Autodesk Inventor part; units mm, degrees
ref_plane "YZ Plane" through (0, 0, 0) normal (1, 0, 0) x (0, 1, 0)
ref_plane "XZ Plane" through (0, 0, 0) normal (0, 1, 0) x (-1, 0, 0)
ref_plane "XY Plane" through (0, 0, 0) normal (0, 0, 1) x (1, 0, 0)
sketch "Sketch1" plane through (0, 0, 0) normal (0, 0, 1) x (1, 0, 0)
  line L0 (0, 0) -> (25, 0)
  line L1 (25, 0) -> (25, 40)
  line L2 (25, 40) -> (0, 40)
  line L3 (0, 40) -> (0, 0)
  dimension "d1" = 25
  dimension "d2" = 40
  dimension "d3" = 25
extrude "Extrusion1" add sketch "Sketch1" against normal blind 30
sketch "Sketch2" plane through (25, 0, 0) normal (1, 0, 0) x (0, 0, -1)
  line L0 (0, 0) -> (30, 0)
  circle A0 centre (15, 6.56) radius 2.46
extrude "Extrusion2" cut sketch "Sketch2" against normal blind 30
sketch "Sketch3" plane through (0, 0, 0) normal (-1, 0, 0) x (0, 0, 1)
  line L0 (0, 0) -> (-30, 0)
  line L1 (-25.05, 0) -> (-4.95, 0)
  line L2 (-4.95, 0) -> (-4.95, 33.12)
  line L3 (-4.95, 33.12) -> (-25.05, 33.12)
  line L4 (-25.05, 33.12) -> (-25.05, 0)
  dimension "d11" = 20.1
extrude "Extrusion3" cut sketch "Sketch3" against normal blind 20
sketch "Sketch4" plane through (0, 0, 0) normal (0, -1, 0) x (1, 0, 0)
  line L0 (20, -4.95) -> (20, -25.05)
  line L1 (20, -15) -> (25, -15)
  line L2 (25, 0) -> (25, -30)
  line L3 (20, -8.025) -> (25, -8.025)
  line L4 (25, -8.025) -> (25, -21.975)
  line L5 (25, -21.975) -> (20, -21.975)
  line L6 (20, -21.975) -> (20, -8.025)
  line L7 (20, -8.025) -> (25, -21.975) construction
  line L8 (25, -8.025) -> (20, -21.975) construction
  line L9 (25, -12.54) -> (25, -17.46)
  point P0 (0, 0)
  point P1 (22.5, -15)
  dimension "d14" = 13.95
extrude "Extrusion4" add sketch "Sketch4" along normal blind 15
sketch "Sketch5" plane through (20, 0, 0) normal (-1, 0, 0) x (0, 0, 1)
  circle A0 centre (-15, 6.56) radius 2.46
  circle A1 centre (-15, 6.56) radius 4.7025
  circle A2 centre (-15, 6.56) radius 2.46
  circle A3 centre (-15, 6.56) radius 2.46
  point P0 (0, 0)
  dimension "d17" = 9.405
extrude "Extrusion5" cut sketch "Sketch5" against normal blind 2.1
sketch "Sketch6" plane through (25, 0, 0) normal (1, 0, 0) x (0, 0, -1)
  circle A0 centre (15, 6.56) radius 4.7025
  line L0 (15, 6.56) -> (15, 23.56)
  circle A1 centre (15, 23.56) radius 2.46
  point P0 (0, 0)
  dimension "d20" = 17
  dimension "d21" = 4.92
extrude "Extrusion6" cut sketch "Sketch6" against normal blind 10 contours A1
sketch "Sketch7" plane through (20, 0, 0) normal (-1, 0, 0) x (0, 0, 1)
  circle A0 centre (-15, 23.56) radius 2.46
  circle A1 centre (-15, 23.56) radius 4.7025
  point P0 (0, 0)
  dimension "d24" = 9.405
extrude "Extrusion7" cut sketch "Sketch7" against normal blind 2.1
sketch "Sketch9" plane through (25, 0, 0) normal (1, 0, 0) x (0, 0, -1)
  circle A0 centre (15, 6.56) radius 2.46
  circle A1 centre (15, 6.56) radius 2.46
  circle A2 centre (15, 23.56) radius 2.46
  circle A3 centre (15, 23.56) radius 2.46
  line L0 (30, 40) -> (30, 0)
  line L1 (30, 0) -> (30, 40)
  line L2 (30, 40) -> (0, 40)
  line L3 (0, 40) -> (0, 0)
  line L4 (0, 0) -> (8.025, 0)
  line L5 (21.975, 0) -> (21.975, -15)
  line L6 (21.975, -15) -> (8.025, -15)
  line L7 (8.025, -15) -> (8.025, 0)
  line L8 (0, 0) -> (8.025, 0)
  line L9 (21.975, 0) -> (30, 0)
extrude "Extrusion8" add sketch "Sketch9" along normal blind 5
sketch "Sketch10" plane through (0, 40, 0) normal (0, 1, 0) x (1, 0, 0)
  line L0 (0, 30) -> (30, 30)
  line L1 (30, 0) -> (0, 0)
  line L2 (0, 30) -> (30, 30)
  line L3 (30, 30) -> (30, 0)
  line L4 (30, 0) -> (0, 0)
  line L5 (0, 0) -> (0, 30)
extrude "Extrusion9" add sketch "Sketch10" along normal blind 30
sketch "Sketch12" plane through (30, 0, 0) normal (1, 0, 0) x (0, 0, -1)
  circle A0 centre (15, 6.56) radius 2.46
  line L0 (15, 6.56) -> (15, 15.06)
  circle A1 centre (15, 15.06) radius 2.525
  point P0 (0, 0)
  dimension "d31" = 8.5
  dimension "d33" = 5.05
extrude "Extrusion10" cut sketch "Sketch12" against normal blind 30 contours A1
sketch "Sketch14" plane through (0, 0, 0) normal (0, 0, 1) x (1, 0, 0)
  line L0 (30, 70) -> (0, 70)
  line L1 (0, 70) -> (0, 85)
  line L2 (-15, 100) -> (-23, 100)
  line L3 (30, 0) -> (30, 70)
  line L4 (30, 113) -> (30, 70)
  arc A0 (0, 85) -> (-15, 100) centre (-15, 85) ccw
  line L5 (30, 105) -> (30, 100)
  line L6 (-23, 128) -> (15, 128)
  line L7 (30, 113) -> (15, 128)
  line L8 (-23, 128) -> (-23, 100)
  point P0 (0, 0)
  point P1 (0, 100)
  dimension "d47" = 30
  dimension "d54" = 15
  dimension "d69" = 28
extrude "Extrusion12" add sketch "Sketch14" against normal blind 30
sketch "Sketch15" plane through (0, 0, -25.05) normal (-1, 0, 0) x (0, 0, 1)
  line L0 (0, 33.12) -> (20.1, 33.12)
  line L1 (20.1, 33.12) -> (20.1, 0)
  line L2 (0, 33.12) -> (20.1, 33.12)
  line L3 (20.1, 33.12) -> (20.1, 31.1)
  line L4 (20.1, 31.1) -> (0, 31.1)
  line L5 (0, 31.1) -> (0, 33.12)
  point P0 (25.05, 0)
  dimension "d57" = 2.02
extrude "Extrusion13" add sketch "Sketch15" against normal blind 20
sketch "Sketch23" plane through (-23, 128, 0) normal (0, 1, 0) x (1, 0, 0)
  line L0 (0, 0) -> (0, 30)
  line L1 (0, 15) -> (0, 2.5)
  line L2 (0, 27.5) -> (0, 15)
  line L3 (0, 27.5) -> (5, 15)
  line L4 (5, 15) -> (0, 2.5)
  point P0 (23, 0)
  dimension "d87" = 12.5
extrude "Extrusion16" cut sketch "Sketch23" against normal through all
properties part number "orien_b_20mm"
Model file for the job. Use its own axes, mm. A direction names the side the tool comes from. Give positions to 0.01 mm unless a question says otherwise; leave off trailing zeros. Loops run counter-clockwise (first coordinate to the right, second up) from the corner with the lowest first, then second, coordinate; pieces in that order, holes last. Notation, with made-up numbers: (33, 31) -> (40, 31) arc R20 ccw to (40, 59) -> close; hole circle Ø8 at (36.5, 11). An arc over 180 degrees is marked (long way). Use a Markdown table: item, result. Add a question column.
(1) Slice it at A-A on y = 15.06. List the corners of the cut face in (x, z) (3 decimals), and give its area (4 significant figures).
(2) Drop flat-ended pins along their axis: pin 1 Ø15 at (y, z) = (35.5, -14.5) entering from -X; pin 2 Ø11 at (x, y) = (24.5, -7.5) entering from -Z (3 decimals); pin 3 Ø2.5 at (x, z) = (13, -27) entering from -Y. Give the stop position or say it passes through.
(3) Mould opens along Z. For faces 1 (the flat face through (10, 31.1, -15)), 2 (the flat face through (18, 0, -27)), 3 (the flat face through (25, -8, -8.025)), 4 (the cylindrical face through (25.07, 15.171, -12.477)) say: +Z half, -Z half, draft (parallel to the pull), parting line (faces both ways), or undercut.
(4) Slice it at D-D on y = 70. List the corners of the cut face in (x, z), and give its area (3 significant figures).
(5) Slice it at C-C on y = -2.5. List the corners of the cut face in (x, z) (3 decimals).
(6) Tool access for faces 5 (the flat face through (-20.465, 114.196, -8.837)), 6 (the cylindrical face through (21.035, 7.973, -10.515)), 7 (the flat face through (10, 16, -25.05)), 8 (the flat face through (-23, 114, -29)), 9 (the flat face through (25, -7, -21.975)): list every direction of +Z, -Z, +X, -X, +Y, -Y with a clear straight run to the whole face (end or side of a thin tool).
(7) Slice it at B-B on x = 3. List the corners of the cut face in (y, z), and give its area (3 significant figures).
(8) Wall check: line 1 along Y through (x, z) = (21.6, -15) (1 decimal); line 2 along Z through (x, y) = (17.5, 6.5); line 3 along Y through (x, z) = (20.8, -15) (1 decimal). Give the ranges that are in metal, low to high.
Filled sheet:
| question | item | result |
|---|---|---|
| 1 | outline | (0, -30) -> (30, -30) -> (30, -17.525) -> (20, -17.525) -> (20, -25.05) -> (0, -25.05) -> close; (0, -4.95) -> (20, -4.95) -> (20, -12.475) -> (30, -12.475) -> (30, 0) -> (0, 0) -> close |
| 1 | area | 447.5 mm2 |
| 2 | pin 1 | x = 0 |
| 2 | pin 2 | z = -21.975 |
| 2 | pin 3 | y = 0 |
| 3 | face 1 | undercut |
| 3 | face 2 | draft |
| 3 | face 3 | +Z half |
| 3 | face 4 | undercut |
| 4 | outline | (0, -30) -> (30, -30) -> (30, 0) -> (0, 0) -> close |
| 4 | area | 900 mm2 |
| 5 | outline | (20, -21.975) -> (30, -21.975) -> (30, -8.025) -> (20, -8.025) -> close |
| 6 | face 5 | -X, +Y, -Y |
| 6 | face 6 | -X |
| 6 | face 7 | -X, -Y |
| 6 | face 8 | +Z, -Z, -X, +Y, -Y |
| 6 | face 9 | -Z, +X, -X, -Y |
| 7 | outline | (0, -30) -> (128, -30) -> (128, 0) -> (0, 0) -> (0, -4.95) -> (31.1, -4.95) -> (31.1, -25.05) -> (0, -25.05) -> close |
| 7 | area | 3,210 mm2 |
| 8 | line 1 | -15 to 1.9, 11.3 to 12.5, 17.6 to 18.9, 28.3 to 121.4 |
| 8 | line 2 | -30 to -25.05, -4.95 to 0 |
| 8 | line 3 | -15 to 1.9, 11.3 to 12.5, 17.6 to 18.9, 28.3 to 122.2 |
